For this review, take the finished solid that the model builds, in its own axes (mm). A direction names the side the tool comes from. Give positions to 0.01 mm unless a question says otherwise; leave off trailing zeros. Write each loop counter-clockwise with the first axis right and the second up, starting at its lowest first coordinate (ties: lowest second). Pieces come first, ordered by that corner, then holes. Notation, with made-up numbers: M 14,23 L 49,23 A25 cw 49,61 Z; hole C 61,23.5 d8. An arc over 180 degrees is marked long. Write item = value, one per line.
```python
from build123d import *

# Parameters (mm, degrees)
CHAPALATERAL_DEPTH        = 380
MOTORTRASEIRO_DEPTH       = 707.113305355
MOTORTRASEIRO_DEPTH_BACK  = 707.113305355
ESBO_O8_W                 = 59.5
ESBO_O8_H                 = 29.2
MOTORFRONTAL_DEPTH        = 707.113305355
MOTORFRONTAL_DEPTH_BACK   = 707.113305355
ESBO_O10_W                = 59.5
ESBO_O10_H                = 29.2
FUROSDYNAMIXEL_DEPTH      = 711.492786733
FUROSDYNAMIXEL_DEPTH_BACK = 711.492786733
ESBO_O15_R                = 1.025


with BuildPart() as part:
    # Chapa inferior → ChapaLateral (new body)
    with BuildSketch(Plane(origin=(0, 0, 0), x_dir=(1, 0, 0), z_dir=(0, 1, 0))):
        with BuildLine():
            Line((-160, 300), (160, 300))
            ThreePointArc((160, 300), (230.710678119, 270.710678119), (260, 200))
            Line((260, 200), (260, -200))
            ThreePointArc((260, -200), (230.710678119, -270.710678119), (160, -300))
            Line((160, -300), (-160, -300))
            ThreePointArc((-160, -300), (-230.710678119, -270.710678119), (-260, -200))
            Line((-260, -200), (-260, 200))
            ThreePointArc((-260, 200), (-230.710678119, 270.710678119), (-160, 300))
        make_face()
        with BuildLine():
            Line((-160, 294), (160, 294))
            ThreePointArc((160, 294), (226.468037432, 266.468037432), (254, 200))
            Line((254, 200), (254, -200))
            ThreePointArc((254, -200), (226.468037432, -266.468037432), (160, -294))
            Line((160, -294), (-160, -294))
            ThreePointArc((-160, -294), (-226.468037432, -266.468037432), (-254, -200))
            Line((-254, -200), (-254, 200))
            ThreePointArc((-254, 200), (-226.468037432, 266.468037432), (-160, 294))
        make_face(mode=Mode.SUBTRACT)
    extrude(amount=CHAPALATERAL_DEPTH)

    # Esboço8 → MotorTraseiro (cut, two sides: drawn at the far end of the back side and taken through both)
    with BuildSketch(Plane.ZY.offset(-254).offset(-MOTORTRASEIRO_DEPTH_BACK)):
        with Locations((-155.25, 20.6)):
            Rectangle(ESBO_O8_W, ESBO_O8_H)
    extrude(amount=MOTORTRASEIRO_DEPTH + MOTORTRASEIRO_DEPTH_BACK, mode=Mode.SUBTRACT)

    # Esboço10 → MotorFrontal (cut, two sides: drawn at the far end of the back side and taken through both)
    with BuildSketch(Plane.ZY.offset(-254).offset(-MOTORFRONTAL_DEPTH_BACK)):
        with Locations((155.25, 20.6)):
            Rectangle(ESBO_O10_W, ESBO_O10_H)
    extrude(amount=MOTORFRONTAL_DEPTH + MOTORFRONTAL_DEPTH_BACK, mode=Mode.SUBTRACT)

    # Esboço15 → FurosDynamixel (cut, two sides: drawn at the far end of the back side and taken through both)
    with BuildSketch(Plane.ZY.offset(260).offset(-FUROSDYNAMIXEL_DEPTH_BACK)):
        with Locations((174.5, 38)):
            Circle(ESBO_O15_R)
        with Locations((152.5, 38)):
            Circle(ESBO_O15_R)
        with Locations((130.5, 38)):
            Circle(ESBO_O15_R)
        with Locations((152.5, 3.4)):
            Circle(ESBO_O15_R)
        with Locations((130.5, 3.4)):
            Circle(ESBO_O15_R)
        with Locations((174.5, 3.4)):
            Circle(ESBO_O15_R)
        with Locations((-174.5, 3.4)):
            Circle(ESBO_O15_R)
        with Locations((-130.5, 3.4)):
            Circle(ESBO_O15_R)
        with Locations((-152.5, 3.4)):
            Circle(ESBO_O15_R)
        with Locations((-130.5, 38)):
            Circle(ESBO_O15_R)
        with Locations((-152.5, 38)):
            Circle(ESBO_O15_R)
        with Locations((-174.5, 38)):
            Circle(ESBO_O15_R)
    extrude(amount=FUROSDYNAMIXEL_DEPTH + FUROSDYNAMIXEL_DEPTH_BACK, mode=Mode.SUBTRACT)


solid = part.part
```
1. For line 1 along Y through (x, z) = (255.6, -174.5) (3 decimals); line 2 along Y through (x, z) = (256, 152); line 3 along X through (y, z) = (134, -15.5), list the stretches that pass through material, from the lowest coordinate up. Write a range as from..to.
Responses:
line_1 = 0..2.375, 4.425..6, 35.2..36.975, 39.025..380
line_2 = 0..2.51, 4.29..6, 35.2..37.11, 38.89..380
line_3 = -260..-254, 254..260
2. Machinability: for faces 4 (the face through (229.929, 187.34, -271.484)), 5 (the face through (-225.733, 187.34, 267.195)), which of the approach directions +Z, -Z, +X, -X, +Y, -Y give a long, thin tool a straight path to every point of the face, cutting with its end or side? Answer none if there is none.
Responses:
face_4 = -Z, +X, +Y, -Y
face_5 = +Y, -Y
3. We need section B-B, the plane y = 217.5. Write out the cut boundary in (x, z), then the cut area to 3 significant figures.
Responses:
outline = M -260,-200 A100 ccw -160,-300 L 160,-300 A100 ccw 260,-200 L 260,200 A100 ccw 160,300 L -160,300 A100 ccw -260,200 Z; hole M -254,-200 A94 ccw -160,-294 L 160,-294 A94 ccw 254,-200 L 254,200 A94 ccw 160,294 L -160,294 A94 ccw -254,200 Z
area = 12,300 mm2
4. The part is to be moulded in two halves that separate along Z. For faces 1 (the face through (260, 187, -3)), 2 (the face through (-231.484, 187.34, -269.929)), 3 (the face through (225.733, 187.34, -267.195)), say which applies: +Z half, -Z half, draft (parallel to the pull), parting line (faces both ways), or undercut.
Responses:
face_1 = draft
face_2 = -Z half
face_3 = undercut
5. We need section A-A, the plane z = 42. Write out the cut boundary in (x, y), then the cut area to 3 significant figures.
Responses:
outline = M -260,0 L -254,0 L -254,380 L -260,380 Z; M 254,0 L 260,0 L 260,380 L 254,380 Z
area = 4,560 mm2
6. We need section D-D, the plane x = -72.5. Write out the cut boundary in (y, z), then the cut area to 3 significant figures.
Responses:
outline = M 0,-300 L 380,-300 L 380,-294 L 0,-294 Z; M 0,294 L 380,294 L 380,300 L 0,300 Z
area = 4,560 mm2
7. We need section C-C, the plane z = 141. Write out the cut boundary in (x, y).
Responses:
outline = M -260,0 L -254,0 L -254,6 L -260,6 Z; M -260,35.2 L -254,35.2 L -254,380 L -260,380 Z; M 254,0 L 260,0 L 260,6 L 254,6 Z; M 254,35.2 L 260,35.2 L 260,380 L 254,380 Z
8. Insertion check: P1, Ø1.8, axis at y = 38, z = 174.5, coming from the +X side; P2, Ø8, axis at x = -193, y = 321.5, coming from the -Z side; P3, Ø1.5, axis at x = -188, y = 276.5, coming from the -Z side. Each pin has a flat end and moves straight along its axis. Give the tip position at first contact, or say it passes through.
Responses:
P1 = through
P2 = -295.7
P3 = -296.22
